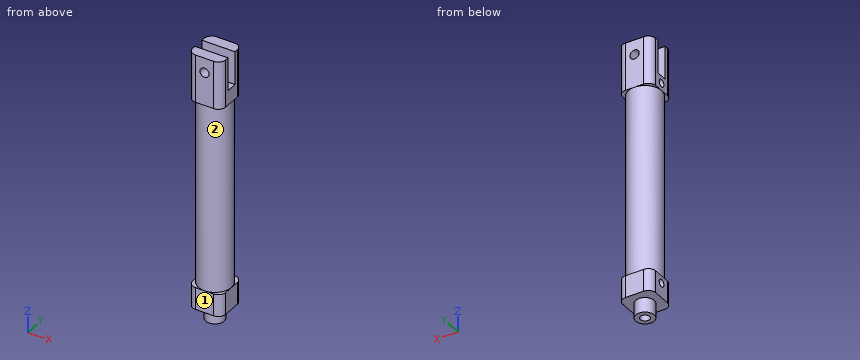
from build123d import *

# Parameters (mm, degrees)
SKETCH_1_R          = 9
SKETCH_1_R_2        = 8
EXTRUDE_1_DEPTH     = 102
EXTRUDE_2_DEPTH     = 26
EXTRUDE_START       = 12
EXTRUDE_3_DEPTH     = 12
SKETCH_4_R          = 5
EXTRUDE_4_DEPTH     = 8
SKETCH_5_R          = 2.5
CUT_EXTRUDE_1_DEPTH = 38
SKETCH_6_R          = 2
SKETCH_6_R_2        = 1.980516498
CUT_EXTRUDE_3_DEPTH = 3
SKETCH_7_W          = 18
SKETCH_7_H          = 6
CUT_EXTRUDE_4_DEPTH = 20
SKETCH_8_R          = 2.5
CUT_EXTRUDE_5_DEPTH = 20


with BuildPart() as part:
    # 草图1 → 凸台-拉伸1 (new body)
    with BuildSketch(Plane.XY):
        Circle(SKETCH_1_R)
        Circle(SKETCH_1_R_2, mode=Mode.SUBTRACT)
    extrude(amount=EXTRUDE_1_DEPTH)

    # 草图2 → 凸台-拉伸2 (add)
    with BuildSketch(Plane.XY.offset(102)):
        with BuildLine():
            Line((-5, -9), (5, -9))
            ThreePointArc((5, -9), (7.828427125, -7.828427125), (9, -5))
            Line((9, -5), (9, 5))
            ThreePointArc((9, 5), (7.828427125, 7.828427125), (5, 9))
            Line((5, 9), (-5, 9))
            ThreePointArc((-5, 9), (-7.828427125, 7.828427125), (-9, 5))
            Line((-9, 5), (-9, -5))
            ThreePointArc((-9, -5), (-7.828427125, -7.828427125), (-5, -9))
        make_face()
    extrude(amount=EXTRUDE_2_DEPTH)

    # 草图3 → 凸台-拉伸3 (add)
    with BuildSketch(Plane(origin=(0, 0, 0), x_dir=(-1, 0, 0), z_dir=(0, 0, -1)).offset(EXTRUDE_START)):
        with BuildLine():
            Line((-5, -9), (5, -9))
            ThreePointArc((5, -9), (7.828427125, -7.828427125), (9, -5))
            Line((9, -5), (9, 5))
            ThreePointArc((9, 5), (7.828427125, 7.828427125), (5, 9))
            Line((5, 9), (-5, 9))
            ThreePointArc((-5, 9), (-7.828427125, 7.828427125), (-9, 5))
            Line((-9, 5), (-9, -5))
            ThreePointArc((-9, -5), (-7.828427125, -7.828427125), (-5, -9))
        make_face()
    extrude(amount=-EXTRUDE_3_DEPTH)

    # 草图4 → 凸台-拉伸4 (add)
    with BuildSketch(Plane(origin=(0, 0, -12), x_dir=(-1, 0, 0), z_dir=(0, 0, -1))):
        Circle(SKETCH_4_R)
    extrude(amount=EXTRUDE_4_DEPTH)

    # 草图5 → 切除-拉伸1 (cut)
    with BuildSketch(Plane(origin=(0, 0, -20), x_dir=(-1, 0, 0), z_dir=(0, 0, -1))):
        Circle(SKETCH_5_R)
    extrude(amount=-CUT_EXTRUDE_1_DEPTH, mode=Mode.SUBTRACT)

    # 草图6 → 切除-拉伸3 (cut)
    with BuildSketch(Plane.ZY.offset(9)):
        with Locations((-4, 0)):
            Circle(SKETCH_6_R)
        with Locations((106, 0)):
            Circle(SKETCH_6_R_2)
    extrude(amount=-CUT_EXTRUDE_3_DEPTH, mode=Mode.SUBTRACT)

    # 草图7 → 切除-拉伸4 (cut)
    with BuildSketch(Plane.ZY.offset(9)):
        with Locations((119, 0)):
            Rectangle(SKETCH_7_W, SKETCH_7_H)
    extrude(amount=-CUT_EXTRUDE_4_DEPTH, mode=Mode.SUBTRACT)

    # 草图8 → 切除-拉伸5 (cut)
    with BuildSketch(Plane.XZ.offset(9)):
        with Locations(Location((0, 120, 0), (0, 0, 270))):
            Circle(SKETCH_8_R)
    extrude(amount=-CUT_EXTRUDE_5_DEPTH, mode=Mode.SUBTRACT)


solid = part.part
CAD build for the part. Positions are in the model's coordinates, mm. Face numbers are marked on the shaded views. Round coordinates to 2 decimals unless told otherwise and drop trailing zeros. Loops run counter-clockwise (first coordinate to the right, second up) from the corner with the lowest first, then second, coordinate; pieces in that order, holes last. Notation, with made-up numbers: (83, 71) - (104, 71) arc R21 ccw to (104, 104) - close; hole circle Ø1 at (41.5, -22.5). An arc over 180 degrees is marked (long way). Put each result on its own line as item: value.
1. Two-plate mould, pull along Z, no slides. Class the marked faces 1 and 2: released by +Z, released by -Z, zero draft, split by the parting line, or undercut.
Geometry check:
face 1: zero draft
face 2: undercut
2. Pin check, flat tips, straight feed: P1, Ø1.5, axis at x = 6, z = 5.5, coming from the -Y side; P2, Ø4.5, axis at x = 6.5, y = 4, coming from the -Z side; P3, Ø2, axis at x = -5, z = 29.5, coming from the +Y side. Stop position of each tip, or through.
Geometry check:
P1: y = -7.31
P2: z = -12
P3: y = 8.06
3. Slice it at A-A on z = 113. List the corners of the cut face in (x, y), and give its area (3 significant figures).
Geometry check:
outline: (-9, -5) arc R4 ccw to (-5, -9) - (5, -9) arc R4 ccw to (9, -5) - (9, -3) - (-9, -3) - close; (-9, 3) - (9, 3) - (9, 5) arc R4 ccw to (5, 9) - (-5, 9) arc R4 ccw to (-9, 5) - close
area: 202 mm²
4. Slice it at B-B on z = -4. List the corners of the cut face in (x, y).
Geometry check:
outline: (-9, -5) arc R4 ccw to (-5, -9) - (5, -9) arc R4 ccw to (9, -5) - (9, 5) arc R4 ccw to (5, 9) - (-5, 9) arc R4 ccw to (-9, 5) - (-9, 2) - (-6, 2) - (-6, -2) - (-9, -2) - close; hole circle Ø5 at (0, 0)
5. Slice it at C-C on z = 82.5. List the corners of the cut face in (x, y), and give its area (3 significant figures).
Geometry check:
outline: circle Ø18 at (0, 0); hole circle Ø16 at (0, 0)
area: 53.4 mm²
6. Wall check: line 1 (Y direction, x = 0, z = 80.5); line 2 (X direction, y = 0.5, z = 7); line 3 (Y direction, x = -3, z = 112.5). Give the ranges that are in metal, low to high.
Geometry check:
line 1: -9 to -8, 8 to 9
line 2: -8.99 to -7.98, 7.98 to 8.99
line 3: -9 to -3, 3 to 9
